Geometry: final body of the model. Coordinates: model frame, mm. A direction names the side the tool comes from. Give positions to 0.01 mm unless a question says otherwise; leave off trailing zeros. Write each loop counter-clockwise with the first axis right and the second up, starting at its lowest first coordinate (ties: lowest second). Pieces come first, ordered by that corner, then holes. Notation, with made-up numbers: (58.5, 74) -> (85.5, 74) arc R12 cw to (85.5, 89) -> close; hole circle Ø9 at (41.5, 78). An arc over 180 degrees is marked (long way). Answer in a Markdown table with one row per item. Add a question column.
Item 1: Section query A-A on x = 0. Output: boundary loops of the cut face in (y, z), plus the area to 3 significant figures.
Item 2: Material intervals for probe 1 along Z at (x, y) = (0, 6); probe 2 along Y at (x, z) = (3.25, -4.5), sorted ascending. Write a range as from..to.
Item 3: Access query for faces 4 (the flat face through (2.5, 0, 1.2)), 5 (the cylindrical face through (4.858, 4.451, -1.53)). Directions: +Z, -Z, +X, -X, +Y, -Y. A direction counts if a zero-diameter tool reaches every point of the face in a straight line with its end or side. Return the directions, or none.
Item 4: First-contact query: P1, Ø1.5, axis at x = 4, y = 5.5, coming from the -Z side; P2, Ø2, axis at x = 0, y = 4.5, coming from the -Z side; P3, Ø2, axis at y = 1, z = 1.5, coming from the +X side. Flat tips, straight axial feed; report the tip coordinate or a pass-through.
Item 5: Section query B-B on y = 7.5. Output: boundary loops of the cut face in (x, z).
Item 6: Draft query along Y for faces 1 (the flat face through (2, 8, 5)), 2 (the flat face through (-2.5, 9, 1.2)), 3 (the cylindrical face through (-5.994, 8.496, -0.264)). Return one class per face: +Y half, -Y half, draft (parallel to the pull), parting line (faces both ways), or undercut.
```python
from build123d import *

# Parameters (mm, degrees)
CHAMFER1_SIZE = 0.2


with BuildPart() as part:
    # Sketch1 → Revolve1 (revolve)
    with BuildSketch(Plane.XY):
        Polygon((2.5, 0), (2.5, 9), (6, 9), (6, 8), (5.092958179, 8), (5.092958179, 1), (6, 1), (6, 0), align=None)
    revolve(axis=Axis((0, 0, 0), (0, 1, 0)))

    # Chamfer1
    chamfer1_edges = [part.edges().sort_by_distance(p)[0] for p in [
        (-6, 0, 0),
        (-6, 1, 0),
        (-6, 8, 0),
        (-6, 9, 0),
    ]]
    chamfer(chamfer1_edges, length=CHAMFER1_SIZE)


solid = part.part
```
Findings below:
| question | item | result |
|---|---|---|
| 1 | outline | (0, -5.8) -> (0.2, -6) -> (0.8, -6) -> (1, -5.8) -> (1, -5.09) -> (8, -5.09) -> (8, -5.8) -> (8.2, -6) -> (8.8, -6) -> (9, -5.8) -> (9, -2.5) -> (0, -2.5) -> close; (0, 2.5) -> (9, 2.5) -> (9, 5.8) -> (8.8, 6) -> (8.2, 6) -> (8, 5.8) -> (8, 5.09) -> (1, 5.09) -> (1, 5.8) -> (0.8, 6) -> (0.2, 6) -> (0, 5.8) -> close |
| 1 | area | 50.1 mm^2 |
| 2 | probe 1 | z = -5.09..-2.5, 2.5..5.09 |
| 2 | probe 2 | y = 0..1, 8..9 |
| 3 | face 4 | +Z, -Z, +X, -X, -Y |
| 3 | face 5 | none |
| 4 | P1 | stops at z = -3.92 |
| 4 | P2 | stops at z = -5.09 |
| 4 | P3 | stops at x = 5.98 |
| 5 | outline | circle Ø10.19 at (0, 0); hole circle Ø5 at (0, 0) |
| 6 | face 1 | undercut |
| 6 | face 2 | +Y half |
| 6 | face 3 | draft |
